Input: part model. Units: mm. Frame: model coordinates. A direction names the side the tool comes from. Coordinates: 2 decimals unless noted, no trailing zeros. Order: outer loops, then holes, each group sorted by start corner. A loop starts at its lowest first (then second) coordinate and runs counter-clockwise, first axis right, second up. Notation, with made-up numbers: (-29.75, 2.25) - (-10.75, 2.25) arc R29 cw to (-10.75, 41.25) - close; hole circle Ø4 at (73.25, 31). An arc over 180 degrees is marked (long way). One line per question, with ' | ' between items.
from build123d import *

# Parameters (mm, degrees)
SKETCH1_W           = 360
SKETCH1_H           = 60
SKETCH1_R           = 7.1
SKETCH1_R_2         = 1.55
SKETCH1_R_3         = 2.55
BOSS_EXTRUDE1_DEPTH = 4
SKETCH2_W           = 360
SKETCH2_H           = 60
SKETCH2_R           = 2.55
SKETCH2_R_2         = 1.55
SKETCH2_R_3         = 7.6
BOSS_EXTRUDE2_DEPTH = 1
CUT_EXTRUDE1_START  = -4
SKETCH2_3_R         = 2.55
SKETCH2_3_R_2       = 1.55
CUT_EXTRUDE1_DEPTH  = 4


with BuildPart() as part:
    # Sketch1 → Boss-Extrude1 (new body)
    with BuildSketch(Plane.XY):
        with Locations((154.041275094, 0)):
            Rectangle(SKETCH1_W, SKETCH1_H)
        with Locations((308.082550187, -0.2)):
            Circle(SKETCH1_R, mode=Mode.SUBTRACT)
        with Locations((-18.451377883, 22.492652976)):
            Circle(SKETCH1_R_2, mode=Mode.SUBTRACT)
        Circle(SKETCH1_R, mode=Mode.SUBTRACT)
        with Locations((-18.451377883, -22.492652976)):
            Circle(SKETCH1_R_2, mode=Mode.SUBTRACT)
        with Locations((50, 0)):
            Circle(SKETCH1_R, mode=Mode.SUBTRACT)
        with Locations((183, 0)):
            Circle(SKETCH1_R, mode=Mode.SUBTRACT)
        with Locations((106.548622117, -22.492652976)):
            Circle(SKETCH1_R_3, mode=Mode.SUBTRACT)
        with Locations((106.548622117, 22.492652976)):
            Circle(SKETCH1_R_3, mode=Mode.SUBTRACT)
    extrude(amount=-BOSS_EXTRUDE1_DEPTH)

    # Sketch2 → Boss-Extrude2 (add)
    with BuildSketch(Plane(origin=(0, 0, -4), x_dir=(-1, 0, 0), z_dir=(0, 0, -1))):
        with Locations((-154.041275094, 0)):
            Rectangle(SKETCH2_W, SKETCH2_H)
        with Locations((-126.548622117, -22.492652976)):
            Circle(SKETCH2_R, mode=Mode.SUBTRACT)
        with Locations(Location((-106.548622117, -22.492652976, 0), (0, 0, 180))):
            Circle(SKETCH2_R, mode=Mode.SUBTRACT)
        with Locations(Location((18.451377883, -22.492652976, 0), (0, 0, 180))):
            Circle(SKETCH2_R_2, mode=Mode.SUBTRACT)
        Circle(SKETCH2_R_3, mode=Mode.SUBTRACT)
        with Locations((-308.082550187, 0)):
            Circle(SKETCH2_R_3, mode=Mode.SUBTRACT)
        with Locations((-183, 0)):
            Circle(SKETCH2_R_3, mode=Mode.SUBTRACT)
        with Locations((-256.65, 26)):
            Circle(SKETCH2_R_2, mode=Mode.SUBTRACT)
        with Locations((-234.35, 26)):
            Circle(SKETCH2_R_2, mode=Mode.SUBTRACT)
        with Locations((-50, 0)):
            Circle(SKETCH2_R_3, mode=Mode.SUBTRACT)
        with Locations((-126.548622117, 22.492652976)):
            Circle(SKETCH2_R, mode=Mode.SUBTRACT)
        with Locations(Location((-106.548622117, 22.492652976, 0), (0, 0, 180))):
            Circle(SKETCH2_R, mode=Mode.SUBTRACT)
        with Locations(Location((18.451377883, 22.492652976, 0), (0, 0, 180))):
            Circle(SKETCH2_R_2, mode=Mode.SUBTRACT)
    extrude(amount=BOSS_EXTRUDE2_DEPTH)

    # Sketch2<3> → Cut-Extrude1 (cut)
    with BuildSketch(Plane(origin=(0, 0, -4), x_dir=(-1, 0, 0), z_dir=(0, 0, -1)).offset(CUT_EXTRUDE1_START)):
        with Locations((-126.548622117, 22.492652976)):
            Circle(SKETCH2_3_R)
        with Locations((-126.548622117, -22.492652976)):
            Circle(SKETCH2_3_R)
        with Locations((-256.65, 26)):
            Circle(SKETCH2_3_R_2)
        with Locations((-234.35, 26)):
            Circle(SKETCH2_3_R_2)
    extrude(amount=CUT_EXTRUDE1_DEPTH, mode=Mode.SUBTRACT)


solid = part.part
Item 1: Ray query, line 1 (X direction, y = -1, z = -2.55); line 2 (Y direction, x = 256.65, z = -3.3); line 3 (X direction, y = -6.5, z = -4.8). Return the intervals inside material, ascending.
Data:
line 1: -25.96 to -7.03, 7.03 to 42.97, 57.03 to 175.97, 190.03 to 301.03, 315.14 to 334.04 | line 2: -30 to 24.45, 27.55 to 30 | line 3: -25.96 to -3.94, 3.94 to 46.06, 53.94 to 179.06, 186.94 to 304.14, 312.02 to 334.04
Item 2: Section A-A on x = 50. Return the cut outline in (y, z), and give its area (3 significant figures).
Data:
outline: (-30, -5) - (-7.6, -5) - (-7.6, -4) - (-7.1, -4) - (-7.1, 0) - (-30, 0) - close; (7.1, -4) - (7.6, -4) - (7.6, -5) - (30, -5) - (30, 0) - (7.1, 0) - close | area: 228 mm^2
Item 3: Section B-B on z = -1.75. Count the separate pieces of the cut face and the enclosed holes in it, and give its area (3 significant figures).
Data:
separate pieces: 1 | enclosed holes: 12 | area: 20,900 mm^2
Item 4: Access query for faces 3 (the face through (314.64, -2.92, -1.97)), 4 (the face through (42.98, -2.91, -4.49)). Directions: +Z, -Z, +X, -X, +Y, -Y. A direction counts if a zero-diameter tool reaches every point of the face in a straight line with its end or side. Return the directions, or none.
Data:
face 3: +Z, -Z | face 4: -Z
Item 5: Draft query along Y for faces 1 (the face through (175.75, 2.28, -4.49)), 2 (the face through (152, 0, 0)). Return one class per face: released by +Y, released by -Y, zero draft, split by the parting line, or undercut.
Data:
face 1: undercut | face 2: zero draft
